```python
from build123d import *

# Parameters (mm, degrees)
EXTRUDE_1_DEPTH     = 585
CUT_EXTRUDE_1_DEPTH = 350
SKETCH_3_R          = 15
CUT_EXTRUDE_2_DEPTH = 591.719899783


with BuildPart() as part:
    # 草图1 → 凸台-拉伸1 (new, symmetric)
    with BuildSketch(Plane.XY):
        with BuildLine():
            Line((-30, 0), (30, 0))
            ThreePointArc((30, 0), (44.142135624, -5.857864376), (50, -20))
            Line((50, -20), (50, -65))
            Line((50, -65), (40, -65))
            Line((40, -65), (40, -20))
            ThreePointArc((40, -20), (37.071067812, -12.928932188), (30, -10))
            Line((30, -10), (-30, -10))
            ThreePointArc((-30, -10), (-37.071067812, -12.928932188), (-40, -20))
            Line((-40, -20), (-40, -65))
            Line((-40, -65), (-50, -65))
            Line((-50, -65), (-50, -20))
            ThreePointArc((-50, -20), (-44.142135624, -5.857864376), (-30, 0))
        make_face()
    extrude(amount=EXTRUDE_1_DEPTH, both=True)

    # 草图2 → 切除-拉伸1 (cut, symmetric)
    with BuildSketch(Plane(origin=(0, 0, 0), x_dir=(0, 0, -1), z_dir=(1, 0, 0))):
        Polygon((-585, -35), (-585, -65), (-562.5, -65), align=None)
        Polygon((562.5, -65), (585, -35), (585, -65), align=None)
    extrude(amount=CUT_EXTRUDE_1_DEPTH, both=True, mode=Mode.SUBTRACT)

    # 草图3 → 切除-拉伸2 (cut, through all)
    with BuildSketch(Plane(origin=(0, 0, 0), x_dir=(1, 0, 0), z_dir=(0, 1, 0))):
        with Locations(Location((0, 522.5, 0), (0, 0, 270))):
            Circle(SKETCH_3_R)
        with Locations(Location((0, -522.5, 0), (0, 0, 270))):
            Circle(SKETCH_3_R)
    extrude(amount=-CUT_EXTRUDE_2_DEPTH, mode=Mode.SUBTRACT)


solid = part.part
```
The model under review builds one solid part; all positions refer to its coordinate system, in mm. A direction names the side the tool comes from. Round coordinates to 2 decimals unless told otherwise and drop trailing zeros. Order: outer loops, then holes, each group sorted by start corner. A loop starts at its lowest first (then second) coordinate and runs counter-clockwise, first axis right, second up.
(1) Tool access review of faces 5 (the face through (-50, -43, 8)), 6 (the face through (0, -10, 8)): name each direction out of +Z, -Z, +X, -X, +Y, -Y from which nothing blocks a thin tool from reaching the whole face with its end or side.
Working result:
face 5: +Z, -Z, -X, +Y, -Y
face 6: +Z, -Z, -Y
(2) For P1, Ø18, axis at x = -1.5, z = 92, coming from the -Y side; P2, Ø5, axis at x = 34.5, z = -120.5, coming from the +Y side; P3, Ø10, axis at x = -26.5, z = 157.5, coming from the -Y side, all flat-tipped, find the tip position at first contact; note any pin that passes through.
Working result:
P1: stops at y = -10
P2: stops at y = -0.1
P3: stops at y = -10.11
(3) Take a section at B-B, the plane x = 0. State the section outline as (y, z) points, plus the area to 3 significant figures.
Working result:
outline: (-10, -585) - (0, -585) - (0, -537.5) - (-10, -537.5) - close; (-10, -507.5) - (0, -507.5) - (0, 507.5) - (-10, 507.5) - close; (-10, 537.5) - (0, 537.5) - (0, 585) - (-10, 585) - close
area: 11,100 mm2
(4) Take a section at C-C, the plane z = -216. State the section outline as (x, y) points, plus the area to 3 significant figures.
Working result:
outline: (-50, -65) - (-40, -65) - (-40, -20) arc R10 cw to (-30, -10) - (30, -10) arc R10 cw to (40, -20) - (40, -65) - (50, -65) - (50, -20) arc R20 ccw to (30, 0) - (-30, 0) arc R20 ccw to (-50, -20) - close
area: 1,970 mm2
(5) Mouldability with a two-part tool opening along X and no side actions: class faces 1 (the face through (1, -9, 585)), 2 (the face through (43.986, -5.703, 8.19)), 3 (the face through (-5.745, -4.93, -508.644)), 4 (the face through (40, -43, 8)) as released by +X, released by -X, zero draft, split by the parting line, or undercut.
Working result:
face 1: zero draft
face 2: released by +X
face 3: undercut
face 4: undercut
(6) Wall thickness on L1, parallel to X at y = -60, z = -41; L2, parallel to Y at x = 26.5, z = 114; L3, parallel to X at y = -17, z = -83: over which ranges is each line inside the solid? List them lowest first.
Working result:
L1: x = -50 to -40, 40 to 50
L2: y = -10 to 0
L3: x = -49.77 to -39.54, 39.54 to 49.77
(7) Take a section at A-A, the plane z = 522.5. State the section outline as (x, y) points, plus the area to 3 significant figures.
Working result:
outline: (-50, -65) - (-40, -65) - (-40, -20) arc R10 cw to (-30, -10) - (-15, -10) - (-15, 0) - (-30, 0) arc R20 ccw to (-50, -20) - close; (15, -10) - (30, -10) arc R10 cw to (40, -20) - (40, -65) - (50, -65) - (50, -20) arc R20 ccw to (30, 0) - (15, 0) - close
area: 1,670 mm2
